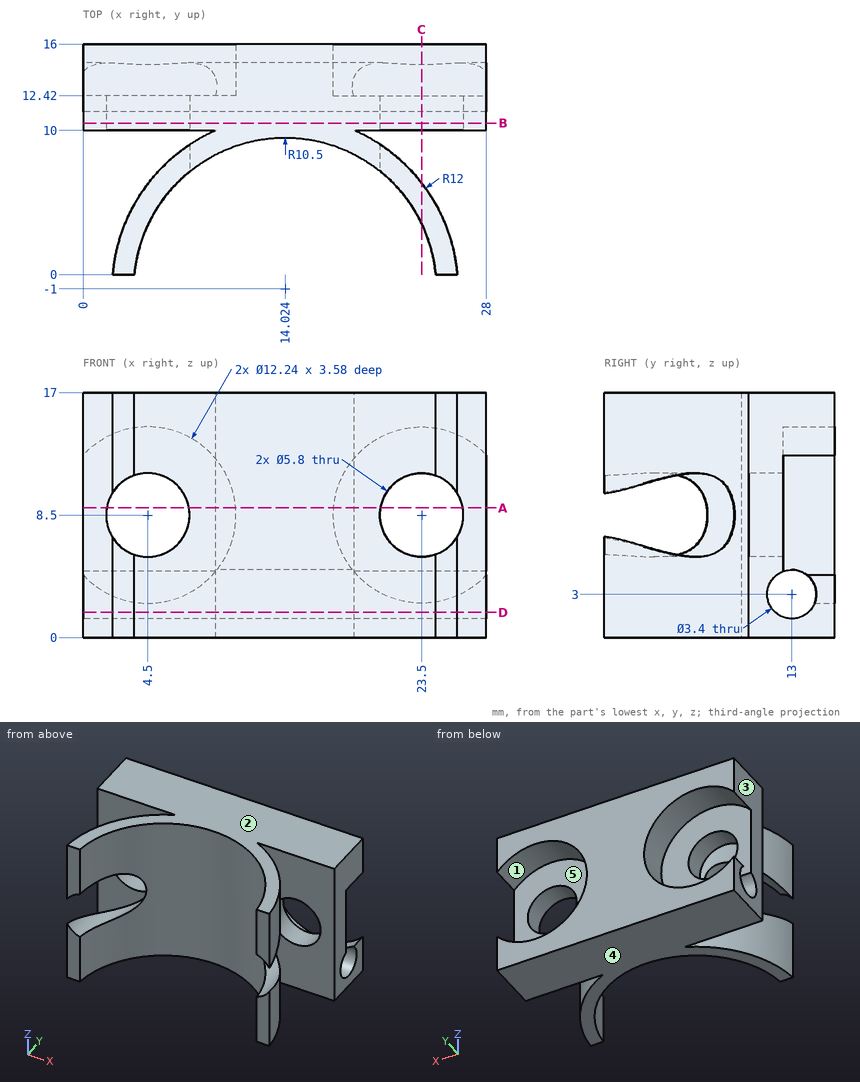
Could you check a few things on this drawing? It's one solid part, dimensions in mm from its lowest x, y, z. A direction names the side the tool comes from. Round coordinates to 2 decimals unless told otherwise and drop trailing zeros. Write each loop counter-clockwise with the first axis right and the second up, starting at its lowest first coordinate (ties: lowest second). Pieces come first, ordered by that corner, then holes. Notation, with made-up numbers: (48.5, 75.5) -> (84.5, 75.5) arc R36 ccw to (84.5, 109.5) -> close; hole circle Ø8 at (-5.75, -30). An arc over 180 degrees is marked (long way). One line per item, written item: value.
1) Suppose I cut it at C-C on x = 23.5. List the corners of the cut face in (y, z) for me.
Filled sheet:
outline: (3.52, 0) -> (6.36, 0) -> (6.36, 5.6) -> (3.52, 5.6) -> close; (3.52, 11.4) -> (6.36, 11.4) -> (6.36, 17) -> (3.52, 17) -> close; (10, 0) -> (16, 0) -> (16, 2.38) -> (14.58, 2.38) arc R1.7 cw (long way) to (12.42, 4.6) -> (12.42, 5.6) -> (10, 5.6) -> close; (10, 11.4) -> (12.42, 11.4) -> (12.42, 14.62) -> (16, 14.62) -> (16, 17) -> (10, 17) -> close
2) Suppose I cut it at D-D on z = 1.75. List the corners of the cut face in (x, y) for me (1 decimal), plus the area to 3 significant figures.
Filled sheet:
outline: (0, 10) -> (9.2, 10) arc R12 ccw to (2.1, 0) -> (3.6, 0) arc R10.5 cw to (24.5, 0) -> (26, 0) arc R12 ccw to (18.8, 10) -> (28, 10) -> (28, 11.8) -> (0, 11.8) -> close; (0, 14.2) -> (28, 14.2) -> (28, 16) -> (0, 16) -> close
area: 147 mm2
3) We'd pull the mould along Z, two halves only. Please class the marked faces 1, 2 and 3: released by +Z, released by -Z, zero draft, split by the parting line, or undercut.
Filled sheet:
face 1: undercut
face 2: released by +Z
face 3: zero draft
4) If I drill on line 1 (Y direction, x = 1.25, z = 3); line 2 (Y direction, x = 20.25, z = 2) (1 decimal); line 3 (X direction, y = 11.25, z = 9), over which ranges is the centre line in solid material (lowest first)? Write a range as [from, to].
Filled sheet:
line 1: y = [10, 11.3], [14.7, 16]
line 2: y = [7.5, 9.3], [10, 11.6], [14.4, 16]
line 3: x = [0, 1.64], [7.36, 20.64], [26.36, 28]
5) I'm going to push flat-ended pins straight in: pin 1 Ø2 at (x, z) = (8.5, 6.5) entering from -Y; pin 2 Ø1.5 at (x, z) = (25, 11) entering from +Y; pin 3 Ø4.5 at (x, z) = (23.5, 8.5) entering from +Y; pin 4 Ø5 at (x, z) = (21, 3) entering from -Y (1 decimal). Where does each tip first touch, or does it pass through?
Filled sheet:
pin 1: stops at y = 7.23
pin 2: stops at y = 12.42
pin 3: passes through
pin 4: stops at y = 3.5
6) For the marked faces 4 and 5, which set-ups out of +Z, -Z, +X, -X, +Y, -Y let a thin tool reach every point of the face, with its end or its side?
Filled sheet:
face 4: -Z, +X, -X, +Y, -Y
face 5: +Y
7) Suppose I cut it at A-A on z = 9. List the corners of the cut face in (x, y) for me (1 decimal).
Filled sheet:
outline: (0, 10) -> (1.6, 10) -> (1.6, 12.4) -> (0, 12.4) -> close; (7.4, 7.1) arc R10.5 cw to (20.6, 7.2) -> (20.6, 9) arc R12 ccw to (18.8, 10) -> (20.6, 10) -> (20.6, 12.4) -> (17.4, 12.4) -> (17.4, 16) -> (10.6, 16) -> (10.6, 12.4) -> (7.4, 12.4) -> (7.4, 10) -> (9.2, 10) arc R12 ccw to (7.4, 9) -> close; (26.4, 10) -> (28, 10) -> (28, 12.4) -> (26.4, 12.4) -> close
8) Suppose I cut it at B-B on y = 10.5. List the corners of the cut face in (x, z) for me, plus the area to 3 significant figures.
Filled sheet:
outline: (0, 0) -> (28, 0) -> (28, 17) -> (0, 17) -> close; hole circle Ø5.8 at (4.5, 8.5); hole circle Ø5.8 at (23.5, 8.5)
area: 423 mm2
